from build123d import *

# Parameters (mm, degrees)
EXTRUDE_THIN1_DEPTH = 1270
FILLET1_R           = 1.27


with BuildPart() as part:
    # Sketch1 → Extrude-Thin1 (new body)
    with BuildSketch(Plane.XY):
        with BuildLine():
            Line((0, 123.03125), (0, 127))
            Line((0, 127), (-36.5125, 127))
            Line((-36.5125, 127), (-36.5125, 114.3))
            Line((-36.5125, 114.3), (-34.13125, 114.3))
            ThreePointArc((-34.13125, 114.3), (-32.654718449, 106.700591974), (-28.1616931, 100.396317948))
            ThreePointArc((-28.1616931, 100.396317948), (-23.520818179, 93.737441229), (-22.225, 85.725))
            Line((-22.225, 85.725), (-19.84375, 85.725))
            Line((-19.84375, 85.725), (-19.84375, 31.75))
            Line((-19.84375, 31.75), (-17.4625, 31.75))
            Line((-17.4625, 31.75), (-17.4625, 12.7))
            Line((-17.4625, 12.7), (-15.08125, 12.7))
            ThreePointArc((-15.08125, 12.7), (-12.058958098, 5.403541902), (-4.7625, 2.38125))
            Line((-4.7625, 2.38125), (-4.7625, 0))
            Line((-4.7625, 0), (0, 0))
            Line((0, 0), (0, 5.55625))
            Line((0, 5.55625), (-1.27, 5.55625))
            Line((-1.27, 5.55625), (-1.27, 1.27))
            Line((-1.27, 1.27), (-3.4925, 1.27))
            Line((-3.4925, 1.27), (-3.4925, 3.740816077))
            ThreePointArc((-3.4925, 3.740816077), (-11.160932486, 6.301567514), (-13.721683923, 13.97))
            Line((-13.721683923, 13.97), (-16.1925, 13.97))
            Line((-16.1925, 13.97), (-16.1925, 33.02))
            Line((-16.1925, 33.02), (-18.57375, 33.02))
            Line((-18.57375, 33.02), (-18.57375, 86.995))
            Line((-18.57375, 86.995), (-20.918106783, 86.995))
            ThreePointArc((-20.918106783, 86.995), (-22.60788254, 94.835880545), (-27.307266754, 101.335921917))
            ThreePointArc((-27.307266754, 101.335921917), (-31.732733484, 107.803797872), (-32.783580599, 115.57))
            Line((-32.783580599, 115.57), (-35.2425, 115.57))
            Line((-35.2425, 115.57), (-35.2425, 125.73))
            Line((-35.2425, 125.73), (-1.27, 125.73))
            Line((-1.27, 125.73), (-1.27, 123.03125))
            Line((-1.27, 123.03125), (0, 123.03125))
        make_face()
    extrude(amount=-EXTRUDE_THIN1_DEPTH)

    # Fillet1
    fillet1_edges = [part.edges().sort_by_distance(p)[0] for p in [
        (-32.783580599, 115.57, -635),
        (-18.57375, 86.995, -635),
        (-16.1925, 33.02, -635),
        (-13.721683923, 13.97, -635),
        (-3.4925, 3.740816077, -635),
        (0, 0, -635),
        (-4.7625, 0, -635),
        (-17.4625, 12.7, -635),
        (-19.84375, 31.75, -635),
        (-22.225, 85.725, -635),
        (-36.5125, 114.3, -635),
        (-36.5125, 127, -635),
        (0, 127, -635),
    ]]
    fillet(fillet1_edges, radius=FILLET1_R)


solid = part.part
Source: CAD feature listing. Evaluate the final solid. Frame: model axes, mm. A direction names the side the tool comes from. Round coordinates to 2 decimals unless told otherwise and drop trailing zeros. Write each loop counter-clockwise with the first axis right and the second up, starting at its lowest first coordinate (ties: lowest second). Pieces come first, ordered by that corner, then holes. Notation, with made-up numbers: M 22,18 L 41,18 A8 ccw 41,28 Z; hole C 7,66 d11. An arc over 180 degrees is marked long. One line per item, written item: value. Start each with the question number.
Item 1: Set-up query: faces 4 (the flat face through (-18.574, 59, -626)), 5 (the flat face through (-19.69, 63.8, 0)), 6 (the flat face through (-19.844, 60, -626)). Return all of +Z, -Z, +X, -X, +Y, -Y with unobstructed straight access to the full face (end or side cutting, diameter ignored); none if empty.
Item 2: Section query A-A (y = 74). Return the cut outline in (x, z).
Item 3: Pin query (flat end, axial travel): pin 1 (16 mm diameter, centred on y = 68, z = -665.5, fed in from +X); pin 2 (19.5 mm diameter, centred on y = 26, z = -794.5, fed in from +X); pin 3 (4 mm diameter, centred on x = -17, y = 73.5, fed in from -Z); pin 4 (2 mm diameter, centred on y = 96.5, z = -321, fed in from +X). Return the tip coordinate at first contact, or that it passes through.
Item 4: Mould query, pull axis Y, two halves, no side actions, for faces 1 (the flat face through (-19.69, 63.8, -1270)), 2 (the flat face through (-18, 127, -626)), 3 (the flat face through (-18, 125.73, -626)). Classes: pulls with the +Y half, pulls with the -Y half, needs draft (parallel to the pull), parting line crosses it, or undercut.
Item 5: Ray query, L1, parallel to Y at x = -20.5, z = -607 (3 decimals); L2, parallel to Y at x = -5, z = -128; L3, parallel to X at y = 64, z = -319. Return the intervals inside material, ascending. Write a range as from..to.
Result set:
1. face 4: +Z, -Z, +X
1. face 5: +Z, +X, -X, +Y, -Y
1. face 6: +Z, -Z, -X, -Y
2. outline: M -19.84,-1270 L -18.57,-1270 L -18.57,0 L -19.84,0 Z
3. pin 1: stops at x = -18.57
3. pin 2: stops at x = -16.19
3. pin 3: stops at z = -1270
3. pin 4: stops at x = -22.92
4. face 1: needs draft
4. face 2: pulls with the +Y half
4. face 3: undercut
5. L1: y = 85.725..86.995, 125.73..127
5. L2: y = 2.38..3.65, 125.73..127
5. L3: x = -19.84..-18.57
